Here's how the part is built. I have some questions about the finished solid (model axes, mm). Face numbers are marked on the shaded views. A direction names the side the tool comes from. Coordinates: 2 decimals unless noted, no trailing zeros. Write each loop counter-clockwise with the first axis right and the second up, starting at its lowest first coordinate (ties: lowest second). Pieces come first, ordered by that corner, then holes.
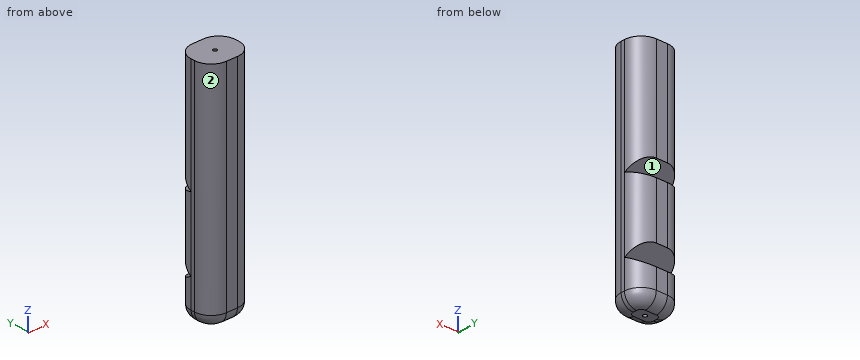
```python
from build123d import *

# Parameters (mm, degrees)
BOSS_EXTRUDE1_DEPTH = 12
SKETCH2_R           = 0.5
CUT_EXTRUDE1_DEPTH  = 63.485196025
FILLET1_R           = 3.25
FILLET2_R           = 4.5


with BuildPart() as part:
    # Sketch1 → Boss-Extrude1 (new body)
    with BuildSketch(Plane(origin=(0, 0, 0), x_dir=(0, 0, -1), z_dir=(1, 0, 0))):
        Polygon((-24.577392289, 0), (35.923845073, 0), (35.923845073, 10), (27.343441845, 10), (25.026106666, 5.553221685), (21.918270736, 10), (7.051101363, 10), (5.673226392, 5.553221685), (2.565390462, 10), (-24.577392289, 10), align=None)
    extrude(amount=BOSS_EXTRUDE1_DEPTH)

    # Sketch2 → Cut-Extrude1 (cut, through all)
    with BuildSketch(Plane.XY.offset(24.577392289)):
        with Locations((6, 5)):
            Circle(SKETCH2_R)
    extrude(amount=-CUT_EXTRUDE1_DEPTH, mode=Mode.SUBTRACT)

    # Fillet1
    fillet1_edges = [part.edges().sort_by_distance(p)[0] for p in [
        (12, 5, -35.923845073),
        (0, 5, -35.923845073),
        (6, 10, -35.923845073),
        (6, 0, -35.923845073),
    ]]
    fillet(fillet1_edges, radius=FILLET1_R)

    # Fillet2
    # the kernel refuses this fillet: 4.5 mm, written as the material it takes off along each edge
    with BuildSketch(Plane(origin=(4.5, 4.5, -35.923845073), x_dir=(0, -1, 0), z_dir=(1, 0, 0))) as fillet2_piece_1:
        with BuildLine():
            CenterArc((1.25, -3.25), 3.25, 0, 90)
            Line((4.5, -3.25), (4.5, 0))
            Line((4.5, 0), (1.25, 0))
        make_face()
    revolve(axis=Axis((4.5, 4.5, -35.923845073), (0, 0, -1)), revolution_arc=90, mode=Mode.SUBTRACT)
    with BuildSketch(Plane(origin=(4.5, 5.5, -35.923845073), x_dir=(-1, 0, 0), z_dir=(0, -1, 0))) as fillet2_piece_2:
        with BuildLine():
            CenterArc((1.25, -3.25), 3.25, 0, 90)
            Line((4.5, -3.25), (4.5, 0))
            Line((4.5, 0), (1.25, 0))
        make_face()
    revolve(axis=Axis((4.5, 5.5, -35.923845073), (0, 0, -1)), revolution_arc=90, mode=Mode.SUBTRACT)
    with BuildSketch(Plane(origin=(7.5, 4.5, -35.923845073), x_dir=(1, 0, 0), z_dir=(0, 1, 0))) as fillet2_piece_3:
        with BuildLine():
            CenterArc((1.25, -3.25), 3.25, 0, 90)
            Line((4.5, -3.25), (4.5, 0))
            Line((4.5, 0), (1.25, 0))
        make_face()
    revolve(axis=Axis((7.5, 4.5, -35.923845073), (0, 0, -1)), revolution_arc=90, mode=Mode.SUBTRACT)
    with BuildSketch(Plane(origin=(7.5, 5.5, -35.923845073), x_dir=(0, 1, 0), z_dir=(-1, 0, 0))) as fillet2_piece_4:
        with BuildLine():
            CenterArc((1.25, -3.25), 3.25, 0, 90)
            Line((4.5, -3.25), (4.5, 0))
            Line((4.5, 0), (1.25, 0))
        make_face()
    revolve(axis=Axis((7.5, 5.5, -35.923845073), (0, 0, -1)), revolution_arc=90, mode=Mode.SUBTRACT)
    with BuildSketch(Plane(origin=(0, 10, -33.168270736), x_dir=(0, -1, 0), z_dir=(0, 0, 1))) as fillet2_piece_5:
        with BuildLine():
            CenterArc((FILLET2_R, FILLET2_R), FILLET2_R, 180, 90)
            Line((0, FILLET2_R), (0, 0))
            Line((0, 0), (FILLET2_R, 0))
        make_face()
    extrude(amount=37.367169374, mode=Mode.SUBTRACT)
    with BuildSketch(Plane(origin=(0, 0, 35.827392289), x_dir=(1, 0, 0), z_dir=(0, 0, -1))) as fillet2_piece_6:
        with BuildLine():
            CenterArc((FILLET2_R, -FILLET2_R), FILLET2_R, 90, 90)
            Line((0, -FILLET2_R), (0, 0))
            Line((0, 0), (FILLET2_R, 0))
        make_face()
    extrude(amount=71.751237362, mode=Mode.SUBTRACT)
    with BuildSketch(Plane(origin=(12, 10, -33.168270736), x_dir=(0, -1, 0), z_dir=(0, 0, 1))) as fillet2_piece_7:
        with BuildLine():
            CenterArc((FILLET2_R, -FILLET2_R), FILLET2_R, 90, 90)
            Line((0, -FILLET2_R), (0, 0))
            Line((0, 0), (FILLET2_R, 0))
        make_face()
    extrude(amount=37.367169374, mode=Mode.SUBTRACT)
    with BuildSketch(Plane(origin=(12, 10, -13.815390462), x_dir=(0, -1, 0), z_dir=(0, 0, 1))) as fillet2_piece_8:
        with BuildLine():
            CenterArc((FILLET2_R, -FILLET2_R), FILLET2_R, 90, 90)
            Line((0, -FILLET2_R), (0, 0))
            Line((0, 0), (FILLET2_R, 0))
        make_face()
    extrude(amount=49.642782751, mode=Mode.SUBTRACT)
    with BuildSketch(Plane(origin=(12, 10, -35.923845073), x_dir=(0, -1, 0), z_dir=(0, 0, 1))) as fillet2_piece_9:
        with BuildLine():
            CenterArc((FILLET2_R, -FILLET2_R), FILLET2_R, 90, 90)
            Line((0, -FILLET2_R), (0, 0))
            Line((0, 0), (FILLET2_R, 0))
        make_face()
    extrude(amount=19.830403228, mode=Mode.SUBTRACT)
    with BuildSketch(Plane(origin=(0, 10, -35.923845073), x_dir=(0, -1, 0), z_dir=(0, 0, 1))) as fillet2_piece_10:
        with BuildLine():
            CenterArc((FILLET2_R, FILLET2_R), FILLET2_R, 180, 90)
            Line((0, FILLET2_R), (0, 0))
            Line((0, 0), (FILLET2_R, 0))
        make_face()
    extrude(amount=19.830403228, mode=Mode.SUBTRACT)
    with BuildSketch(Plane(origin=(12, 0, 35.827392289), x_dir=(-1, 0, 0), z_dir=(0, 0, -1))) as fillet2_piece_11:
        with BuildLine():
            CenterArc((FILLET2_R, FILLET2_R), FILLET2_R, 180, 90)
            Line((0, FILLET2_R), (0, 0))
            Line((0, 0), (FILLET2_R, 0))
        make_face()
    extrude(amount=71.751237362, mode=Mode.SUBTRACT)
    with BuildSketch(Plane(origin=(0, 10, -13.815390462), x_dir=(0, -1, 0), z_dir=(0, 0, 1))) as fillet2_piece_12:
        with BuildLine():
            CenterArc((FILLET2_R, FILLET2_R), FILLET2_R, 180, 90)
            Line((0, FILLET2_R), (0, 0))
            Line((0, 0), (FILLET2_R, 0))
        make_face()
    extrude(amount=49.642782751, mode=Mode.SUBTRACT)


solid = part.part
```
1) Imagine slicing it at A-A on x = 6. Please give me the cut outline in (y, z), then the cut area to 3 significant figures.
Values follow:
outline: (0, -32.67) arc R3.25 ccw to (3.25, -35.92) - (4.5, -35.92) - (4.5, 24.58) - (0, 24.58) - close; (5.5, -35.92) - (6.75, -35.92) arc R3.25 ccw to (10, -32.67) - (10, -27.34) - (5.55, -25.03) - (10, -21.92) - (10, -7.05) - (5.55, -5.67) - (10, -2.57) - (10, 24.58) - (5.5, 24.58) - close
area: 518 mm2
2) Will these pins go through, and if not, where does the flat tip stop? pin 1 (1 mm diameter, centred on y = 7, z = -9, fed in from -X); pin 2 (1.5 mm diameter, centred on x = 10, z = -7.5, fed in from +Y); pin 3 (1 mm diameter, centred on y = 7, z = -4, fed in from +X).
Values follow:
pin 1: stops at x = 0.11
pin 2: stops at y = 9.65
pin 3: stops at x = 11.89
3) I need wall thicknesses on probe 1 along Y at (x, z) = (6, 5); probe 2 along Z at (x, y) = (7.25, 9.25); probe 3 along Z at (x, y) = (7.75, 7). Which ranges of each line are inside material? Lowest first, please.
Values follow:
probe 1: y = 0 to 4.5, 5.5 to 10
probe 2: z = -34.75 to -26.95, -22.44 to -6.82, -3.09 to 24.58
probe 3: z = -35.91 to -25.78, -24.01 to -6.12, -4.66 to 24.58
4) Imagine slicing it at C-C on y = 7.5. Count the separate pieces of the cut face and the enclosed holes in it, then the cut area to 3 significant figures.
Values follow:
separate pieces: 3
enclosed holes: 0
area: 615 mm2
5) On a 3-axis mill with a long thin cutter (end or side, diameter ignored), from which of +Z, -Z, +X, -X, +Y, -Y can I reach the whole of each face in a straight line? I mean the marked faces 1 and 2. Say none if no direction works.
Values follow:
face 1: +X, -X, +Y
face 2: +Z, -Z, -X, -Y
6) Imagine slicing it at B-B on z = -28.5. Please give me the cut outline in (x, y), then the cut area to 3 significant figures.
Values follow:
outline: (0, 4.5) arc R4.5 ccw to (4.5, 0) - (7.5, 0) arc R4.5 ccw to (12, 4.5) - (12, 5.5) arc R4.5 ccw to (7.5, 10) - (4.5, 10) arc R4.5 ccw to (0, 5.5) - close; hole circle Ø1 at (6, 5)
area: 102 mm2
